Source: three-view drawing plus pictorial views. Frame: mm from the lowest corner of the part. Coordinates: 2 decimals unless noted, no trailing zeros. Order: outer loops, then holes, each group sorted by start corner. A loop starts at its lowest first (then second) coordinate and runs counter-clockwise, first axis right, second up. Notation, with made-up numbers: M 20.5,36.25 L 29.5,36.25 A14 ccw 29.5,41.25 Z; hole C -18.5,28.25 d10. An arc over 180 degrees is marked long. One line per question, with ' | ' between items.
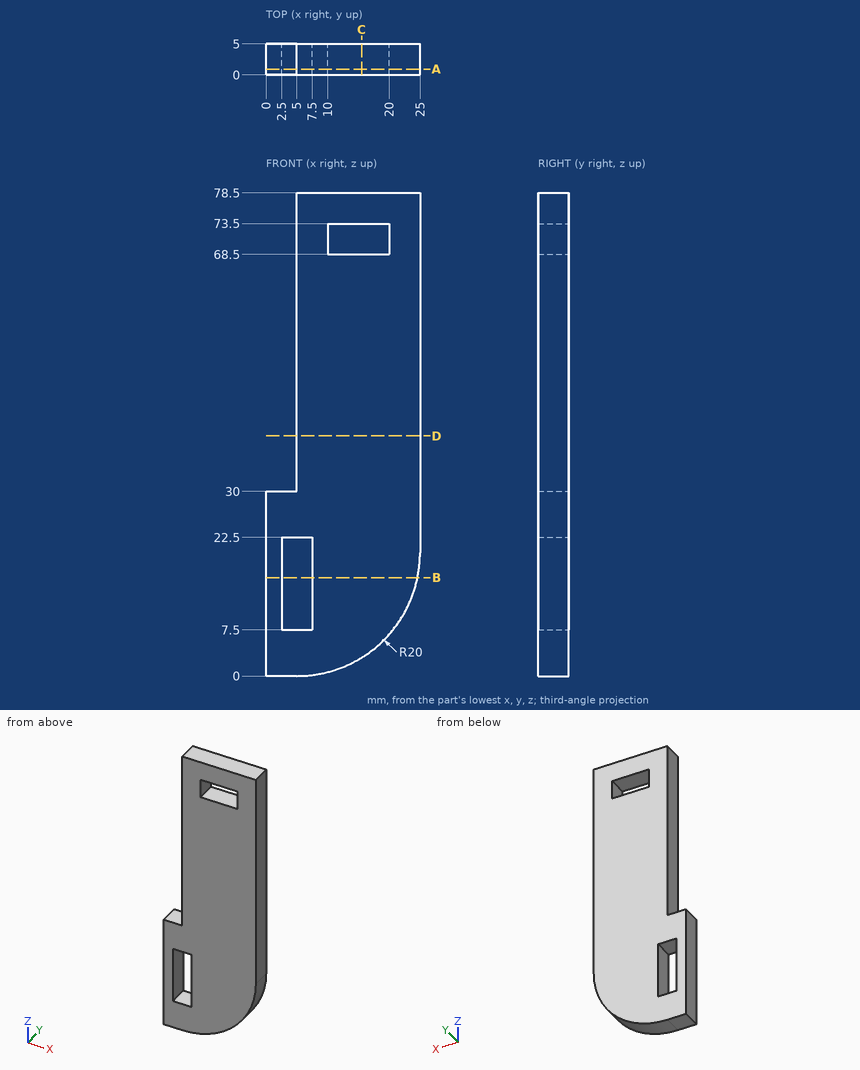
1. Section D-D, the plane z = 39. Output: boundary loops of the cut face in (x, y), and give its area (3 significant figures).
Response values:
outline: M 5,0 L 25,0 L 25,5 L 5,5 Z | area: 100 mm^2
2. Section A-A, the plane y = 0.9. Output: boundary loops of the cut face in (x, z), and give its area (3 significant figures).
Response values:
outline: M 0,0 L 5,0 A20 ccw 25,20 L 25,78.5 L 5,78.5 L 5,30 L 0,30 Z; hole M 2.5,7.5 L 7.5,7.5 L 7.5,22.5 L 2.5,22.5 Z; hole M 10,68.5 L 20,68.5 L 20,73.5 L 10,73.5 Z | area: 1,510 mm^2
3. Section B-B, the plane z = 16. Output: boundary loops of the cut face in (x, y).
Response values:
outline: M 0,0 L 2.5,0 L 2.5,5 L 0,5 Z; M 7.5,0 L 24.6,0 L 24.6,5 L 7.5,5 Z
4. Section C-C, the plane x = 15.5. Output: boundary loops of the cut face in (y, z), and give its area (3 significant figures).
Response values:
outline: M 0,2.98 L 5,2.98 L 5,68.5 L 0,68.5 Z; M 0,73.5 L 5,73.5 L 5,78.5 L 0,78.5 Z | area: 353 mm^2
5. Material intervals for line 1 (X direction, y = 4.4, z = 21); line 2 (X direction, y = 3.65, z = 75.5); line 3 (Z direction, x = 17.5, y = 0.7), sorted ascending. Write a range as [from, to].
Response values:
line 1: x = [0, 2.5], [7.5, 25] | line 2: x = [5, 25] | line 3: z = [4.39, 68.5], [73.5, 78.5]
